Work out the finished part from the listing and answer in its coordinate system (mm). A direction names the side the tool comes from. Coordinates: 2 decimals unless noted, no trailing zeros. Write each loop counter-clockwise with the first axis right and the second up, starting at its lowest first coordinate (ties: lowest second). Pieces come first, ordered by that corner, then holes. Notation, with made-up numbers: (25, -38.5) - (53, -38.5) arc R17 ccw to (53, -24.5) - close; hole circle Ø3 at (-15.5, -24). An arc over 180 degrees is marked (long way). Answer as a JSON object with one key per item and string values. Group by question number.
from build123d import *

# Parameters (mm, degrees)
SKETCH1_W           = 20
SKETCH1_H           = 20
BOSS_EXTRUDE2_DEPTH = 1
SKETCH1_6_W         = 22
SKETCH1_6_H         = 22
SKETCH1_6_W_2       = 20
SKETCH1_6_H_2       = 20
BOSS_EXTRUDE3_DEPTH = 6
SKETCH2_R           = 0.4
BOSS_EXTRUDE4_DEPTH = 0.5
FILLET1_R           = 1.5


with BuildPart() as part:
    # Sketch1 → Boss-Extrude2 (new body)
    with BuildSketch(Plane(origin=(0, 0, 0), x_dir=(1, 0, 0), z_dir=(0, 1, 0))):
        Rectangle(SKETCH1_W, SKETCH1_H)
    extrude(amount=BOSS_EXTRUDE2_DEPTH)

    # Sketch1<6> → Boss-Extrude3 (add)
    with BuildSketch(Plane(origin=(0, 0, 0), x_dir=(1, 0, 0), z_dir=(0, 1, 0))):
        Rectangle(SKETCH1_6_W, SKETCH1_6_H)
        Rectangle(SKETCH1_6_W_2, SKETCH1_6_H_2, mode=Mode.SUBTRACT)
    extrude(amount=BOSS_EXTRUDE3_DEPTH)

    # Sketch2 → Boss-Extrude4 (add)
    with BuildSketch(Plane(origin=(0, 6, 0), x_dir=(1, 0, 0), z_dir=(0, 1, 0))):
        with Locations((0, 10.490155688)):
            Circle(SKETCH2_R)
        with Locations((1, 10.490155688)):
            Circle(SKETCH2_R)
        with Locations((-1, 10.490155688)):
            Circle(SKETCH2_R)
        with Locations((-2, 10.490155688)):
            Circle(SKETCH2_R)
        with Locations((2, 10.490155688)):
            Circle(SKETCH2_R)
    extrude(amount=BOSS_EXTRUDE4_DEPTH)

    # Fillet1
    fillet1_edges = [part.edges().sort_by_distance(p)[0] for p in [
        (10, 3.5, -10),
        (-10, 3.5, -10),
        (-10, 3.5, 10),
        (10, 3.5, 10),
    ]]
    fillet(fillet1_edges, radius=FILLET1_R)


solid = part.part
Q1. Section B-B on z = -7.25 is taken. Determine the outline of the cut face in (x, y), plus the area to 3 significant figures.
Q2. Section D-D on x = 4.25 is taken. Determine the outline of the cut face in (y, z), plus the area to 3 significant figures.
Q3. Consider L1, parallel to Z at x = -6.75, y = 3.5; L2, parallel to Y at x = 9.75, z = -7.5. Determine where each line is inside the solid, lowest interval first. Write a range as from..to.
Q4. A tool of negligible diameter and unlimited length cuts with its end or side. For faces 1 (the face through (0, 3, -11)), 2 (the face through (-10, 3, 0)), from which of +Z, -Z, +X, -X, +Y, -Y can it reach the whole face along a straight path? Write none if from no direction.
Q5. For a pull along X with two mould halves and no side action, classify faces 3 (the face through (0, 3, 11)), 4 (the face through (11, 3, 0)), 5 (the face through (-11, 3, 0)), 6 (the face through (-9.55, 3.54, 9.57)) as +X half, -X half, draft (parallel to the pull), parting line (faces both ways), or undercut.
Q6. Section A-A on x = -2 is taken. Determine the outline of the cut face in (y, z).
Q7. Flat-ended cylindrical pins translate along their axes: pin 1 Ø4 at (x, z) = (5.5, 4.5) entering from +Y; pin 2 Ø4 at (x, z) = (-5.5, -7.5) entering from -Y. Find the tip coordinate at first contact, or state that the pin passes through.
Q8. Section C-C on y = 2.25 is taken. Determine the outline of the cut face in (x, z).
Numbers:
{
 "1": {"outline": "(-11, 0) - (11, 0) - (11, 6) - (10, 6) - (10, 1) - (-10, 1) - (-10, 6) - (-11, 6) - close", "area": "32.0 mm²"},
 "2": {"outline": "(0, -11) - (6, -11) - (6, -10) - (1, -10) - (1, 10) - (6, 10) - (6, 11) - (0, 11) - close", "area": "32.0 mm²"},
 "3": {"L1": "z = -11..-10, 10..11", "L2": "y = 0..1"},
 "4": {"face 1": "-Z, +X, -X, +Y, -Y", "face 2": "+Y"},
 "5": {"face 3": "draft", "face 4": "+X half", "face 5": "-X half", "face 6": "undercut"},
 "6": {"outline": "(0, -11) - (6, -11) - (6, -10.89) - (6.5, -10.89) - (6.5, -10.09) - (6, -10.09) - (6, -10) - (1, -10) - (1, 10) - (6, 10) - (6, 11) - (0, 11) - close"},
 "7": {"pin 1": "stops at y = 1", "pin 2": "stops at y = 0"},
 "8": {"outline": "(-11, -11) - (11, -11) - (11, 11) - (-11, 11) - close; hole (-10, -8.5) arc R1.5 ccw to (-8.5, -10) - (8.5, -10) arc R1.5 ccw to (10, -8.5) - (10, 8.5) arc R1.5 ccw to (8.5, 10) - (-8.5, 10) arc R1.5 ccw to (-10, 8.5) - close"}
}
